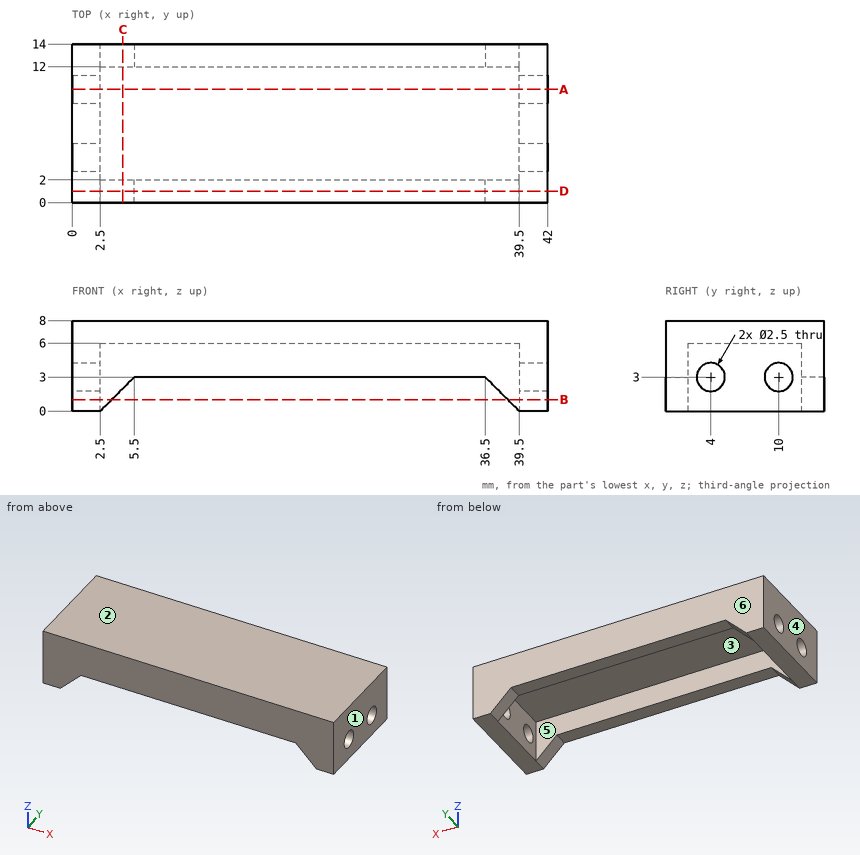
Geometry check sheet. Reference: drawing and pictorial views, mm from the part's lowest x, y, z. A direction names the side the tool comes from. Give positions to 0.01 mm unless a question says otherwise; leave off trailing zeros. Order: outer loops, then holes, each group sorted by start corner. A loop starts at its lowest first (then second) coordinate and runs counter-clockwise, first axis right, second up. Notation, with made-up numbers: (85.5, 62) - (107.5, 62) arc R26 ccw to (107.5, 76) - close; hole circle Ø9 at (-3.5, 3.5). An arc over 180 degrees is marked (long way). Answer as CSV lines item,"result". Start each with the question number.
Item 1: Mould release check, pull along X, two halves, no side actions. Record for the marked faces 1, 2, 3 and 4: released by +X, released by -X, zero draft, split by the parting line, or undercut.
Item 2: Section check C-C, the plane x = 4.5. Record the boundary of the cut face in (y, z).
Item 3: Material ranges on L1, parallel to Y at x = 41.25, z = 3; L2, parallel to X at y = 10.25, z = 1.5; L3, parallel to Z at x = 35.5, y = 7.25, recorded low to high.
Item 4: Gauge pin test, flat ends, axial feed: pin 1 (4 mm diameter, centred on y = 4, z = 3, fed in from +X); pin 2 (1.6 mm diameter, centred on x = 24, y = 0.5, fed in from -Z); pin 3 (8 mm diameter, centred on x = 14.5, y = 6.5, fed in from -Z). Record the tip position at first contact, or that the pin passes through.
Item 5: Access from +Z, -Z, +X, -X, +Y, -Y to the whole of each face (thin tool, end or side, straight path). Record for the marked faces 5 and 6.
Item 6: Section check A-A, the plane y = 10. Record the boundary of the cut face in (x, z), plus the area to 4 significant figures.
Item 7: Section check D-D, the plane y = 1. Record the boundary of the cut face in (x, z).
Item 8: Section check B-B, the plane z = 1. Record the boundary of the cut face in (x, y), plus the area to 3 significant figures.
Filled in:
1,face 1,"released by +X"
1,face 2,"zero draft"
1,face 3,"undercut"
1,face 4,"released by -X"
2,outline,"(0, 2) - (2, 2) - (2, 6) - (12, 6) - (12, 2) - (14, 2) - (14, 8) - (0, 8) - close"
3,L1,"0 to 2.75, 5.25 to 8.75, 11.25 to 14"
3,L2,"0 to 2.5, 39.5 to 42"
3,L3,"6 to 8"
4,pin 1,"x = 42"
4,pin 2,"z = 3"
4,pin 3,"z = 6"
5,face 5,"-Z"
5,face 6,"+Z, -Z, +X, -X, +Y"
6,outline,"(0, 0) - (2.5, 0) - (2.5, 1.75) - (0, 1.75) - close; (0, 4.25) - (2.5, 4.25) - (2.5, 6) - (39.5, 6) - (39.5, 4.25) - (42, 4.25) - (42, 8) - (0, 8) - close; (39.5, 0) - (42, 0) - (42, 1.75) - (39.5, 1.75) - close"
6,area,"101.5 mm^2"
7,outline,"(0, 0) - (2.5, 0) - (5.5, 3) - (36.5, 3) - (39.5, 0) - (42, 0) - (42, 8) - (0, 8) - close"
8,outline,"(0, 0) - (3.5, 0) - (3.5, 2) - (2.5, 2) - (2.5, 12) - (3.5, 12) - (3.5, 14) - (0, 14) - close; (38.5, 0) - (42, 0) - (42, 14) - (38.5, 14) - (38.5, 12) - (39.5, 12) - (39.5, 2) - (38.5, 2) - close"
8,area,"78.0 mm^2"
